Work out the finished part from the listing and answer in its coordinate system (mm). Coordinates: 2 decimals unless noted, no trailing zeros. Order: outer loops, then holes, each group sorted by start corner. A loop starts at its lowest first (then second) coordinate and runs counter-clockwise, first axis right, second up. Notation, with made-up numbers: (1.5, 48) -> (11.5, 48) arc R13 cw to (11.5, 57) -> close; hole circle Ø1 at (64, 38). An arc over 180 degrees is marked (long way). Write item = value, one per line. Start each with the question number.
Q1. The part is cut by section B-B, the plane z = -80.5. Determine the outline of the cut face in (x, y).
Q2. A flat-ended cylindrical pin translates along its axis: pin 1 (10 mm diameter, centred on y = 11, z = -19, fed in from -X). Find the tip coordinate at first contact, or state that the pin passes through.
Q3. Straight lines are drawn through the part: L1, parallel to Y at x = 2.25, z = -88.9; L2, parallel to Y at x = 1.5, z = -31; L3, parallel to Z at x = 1, y = -13. For each, find the intervals that lie inside material, in ascending order. Write a range as from..to.
Q4. The part is cut by section C-C, the plane x = 2. Count the separate pieces of the cut face and the enclosed holes in it, plus the area to 3 significant figures.
Q5. The part is cut by section A-A, the plane y = 0. Determine the outline of the cut face in (x, z), plus the area to 3 significant figures.
Q6. The part is cut by section D-D, the plane y = -16. Determine the outline of the cut face in (x, z).
```python
from build123d import *

# Parameters (mm, degrees)
SKETCH2_R           = 14.2875
SKETCH2_R_2         = 2.0193
BOSS_EXTRUDE1_DEPTH = 6.35


with BuildPart() as part:
    # Sketch2 → Boss-Extrude1 (new body)
    with BuildSketch(Plane(origin=(0, 0, 0), x_dir=(0, 0, -1), z_dir=(1, 0, 0))):
        with BuildLine():
            Line((0, 19.05), (0, -19.05))
            Line((0, -19.05), (88.9, -19.05))
            ThreePointArc((88.9, -19.05), (107.95, 0), (88.9, 19.05))
            Line((88.9, 19.05), (0, 19.05))
        make_face()
        with Locations((88.9, 0)):
            Circle(SKETCH2_R, mode=Mode.SUBTRACT)
        with Locations((3.175, -9.525)):
            Circle(SKETCH2_R_2, mode=Mode.SUBTRACT)
        with Locations((3.175, 9.525)):
            Circle(SKETCH2_R_2, mode=Mode.SUBTRACT)
        with Locations((32.025, -9.525)):
            Circle(SKETCH2_R_2, mode=Mode.SUBTRACT)
        with Locations((32.025, 9.525)):
            Circle(SKETCH2_R_2, mode=Mode.SUBTRACT)
    extrude(amount=BOSS_EXTRUDE1_DEPTH)


solid = part.part
```
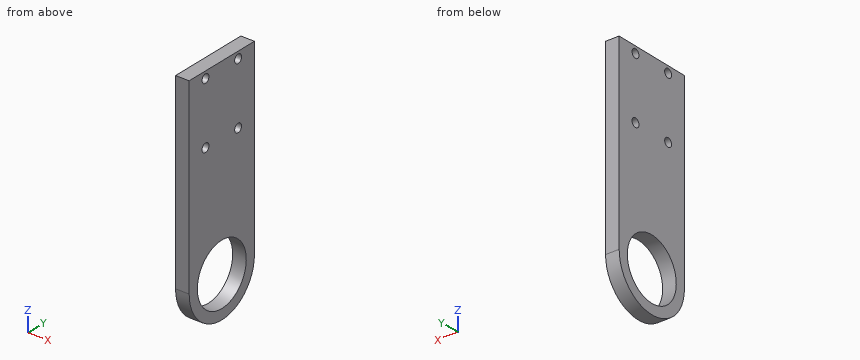
Model answer:
q1.outline = (0, -19.05) -> (6.35, -19.05) -> (6.35, -11.56) -> (0, -11.56) -> close; (0, 11.56) -> (6.35, 11.56) -> (6.35, 19.05) -> (0, 19.05) -> close
q2.pin_1 = 0
q3.L1 = -19.05..-14.29, 14.29..19.05
q3.L2 = -19.05..-11.26, -7.79..7.79, 11.26..19.05
q3.L3 = -102.82..-94.83, -82.97..0
q4.separate_pieces = 1
q4.enclosed_holes = 5
q4.area = 3,260 mm2
q5.outline = (0, -107.95) -> (6.35, -107.95) -> (6.35, -103.19) -> (0, -103.19) -> close; (0, -74.61) -> (6.35, -74.61) -> (6.35, 0) -> (0, 0) -> close
q5.area = 504 mm2
q6.outline = (0, -99.24) -> (6.35, -99.24) -> (6.35, 0) -> (0, 0) -> close
